Source: CAD feature listing. Evaluate the final solid. Frame: model axes, mm. A direction names the side the tool comes from. Round coordinates to 2 decimals unless told otherwise and drop trailing zeros. Order: outer loops, then holes, each group sorted by start corner. A loop starts at its lowest first (then second) coordinate and runs counter-clockwise, first axis right, second up. Notation, with made-up numbers: M -40,32.25 L -31,32.25 A18 cw -31,56.25 Z; hole C 81,45.25 d7. An arc over 180 degrees is marked long. Answer in a Markdown table with one row per item. Add a question column.
```python
from build123d import *

# Parameters (mm, degrees)
SKETCH1_W                     = 28.2
SKETCH1_H                     = 28.2
BOSS_EXTRUDE1_DEPTH           = 49
SKETCH2_R                     = 11
BOSS_EXTRUDE2_DEPTH           = 2
SKETCH3_R                     = 2.5
BOSS_EXTRUDE3_DEPTH           = 18
FILLET1_R                     = 2
TAP_DRILL_FOR_M2_5_TAP1_D     = 2.05
TAP_DRILL_FOR_M2_5_TAP1_DEPTH = 4.5
TAP_DRILL_FOR_M2_5_TAP1_TIP   = 0.615882135
FILLET2_R                     = 1


with BuildPart() as part:
    # Sketch1 → Boss-Extrude1 (new body)
    with BuildSketch(Plane(origin=(0, 0, 0), x_dir=(1, 0, 0), z_dir=(0, 1, 0))):
        with Locations((14.1, 14.1)):
            Rectangle(SKETCH1_W, SKETCH1_H)
    extrude(amount=BOSS_EXTRUDE1_DEPTH)

    # Sketch2 → Boss-Extrude2 (add)
    with BuildSketch(Plane(origin=(0, 49, 0), x_dir=(1, 0, 0), z_dir=(0, 1, 0))):
        with Locations(Location((14.1, 14.1, 0), (0, 0, 270))):
            Circle(SKETCH2_R)
    extrude(amount=BOSS_EXTRUDE2_DEPTH)

    # Sketch3 → Boss-Extrude3 (add)
    with BuildSketch(Plane(origin=(0, 51, 0), x_dir=(1, 0, 0), z_dir=(0, 1, 0))):
        with Locations(Location((14.1, 14.1, 0), (0, 0, 270))):
            Circle(SKETCH3_R)
    extrude(amount=BOSS_EXTRUDE3_DEPTH)

    # Fillet1
    fillet1_edges = [part.edges().sort_by_distance(p)[0] for p in [
        (0, 24.5, -28.2),
        (28.2, 24.5, -28.2),
        (28.2, 24.5, 0),
        (0, 24.5, 0),
    ]]
    fillet(fillet1_edges, radius=FILLET1_R)

    # Tap Drill for M2.5 Tap1
    with Locations(Plane(origin=(0, 49, 0), x_dir=(1, 0, 0), z_dir=(0, 1, 0))):
        with Locations((2.6, 2.6), (25.6, 2.6), (25.6, 25.6), (2.6, 25.6)):
            Hole(TAP_DRILL_FOR_M2_5_TAP1_D / 2, depth=TAP_DRILL_FOR_M2_5_TAP1_DEPTH)
            with Locations((0, 0, -(TAP_DRILL_FOR_M2_5_TAP1_DEPTH + TAP_DRILL_FOR_M2_5_TAP1_TIP / 2))):  # 118° drill point
                Cone(0, TAP_DRILL_FOR_M2_5_TAP1_D / 2, TAP_DRILL_FOR_M2_5_TAP1_TIP, mode=Mode.SUBTRACT)

    # Fillet2
    fillet2_edges = [part.edges().sort_by_distance(p)[0] for p in [
        (14.1, 0, -28.2),
        (0, 0, -14.1),
        (28.2, 0, -14.1),
        (14.1, 0, 0),
        (0.585786438, 0, -0.585786438),
        (27.614213562, 0, -0.585786438),
        (0.585786438, 0, -27.614213562),
        (27.614213562, 0, -27.614213562),
    ]]
    fillet(fillet2_edges, radius=FILLET2_R)


solid = part.part
```
(1) Cut plane A-A (z = -14.1). Return loops of the section in (x, y), and give its area (3 significant figures).
(2) Pin query (flat end, axial travel): pin 1 (2.5 mm diameter, centred on x = 2.6, z = -2.6, fed in from +Y). Return the tip coordinate at first contact, or that it passes through.
(3) Draft query along X for faces 3 (the face through (0.57, 25.34, -0.6)), 4 (the face through (27.6, 25.34, -27.63)), 5 (the face through (24.65, 46.72, -25.21)). Return one class per face: +X half, -X half, draft (parallel to the pull), parting line (faces both ways), or undercut.
(4) Cut plane B-B (x = 6). Return loops of the section in (y, z), and give its area (3 significant figures).
(5) Cut plane C-C (y = 58.5). Return loops of the section in (x, z), and give its area (3 significant figures).
(6) Cut plane D-D (z = -21). Return loops of the section in (x, y).
(7) Access query for faces 1 (the face through (28.2, 25, -14)), 2 (the face through (8, 49, -24)). Directions: +Z, -Z, +X, -X, +Y, -Y. A direction counts if a zero-diameter tool reaches every point of the face in a straight line with its end or side. Return the directions, or none.
(8) Line query: line 1 (Z direction, x = 2.6, y = 47.25) (3 decimals); line 2 (X direction, y = 47.7, z = -25.6) (3 decimals); line 3 (Y direction, x = 14.5, z = -26.75). Output: solid intervals per line, ascending. Write a range as from..to.
Answer list:
| question | item | result |
|---|---|---|
| 1 | outline | M 0,1 A1 ccw 1,0 L 27.2,0 A1 ccw 28.2,1 L 28.2,49 L 25.1,49 L 25.1,51 L 16.6,51 L 16.6,69 L 11.6,69 L 11.6,51 L 3.1,51 L 3.1,49 L 0,49 Z |
| 1 | area | 1,520 mm² |
| 2 | pin 1 | y = 49 |
| 3 | face 3 | -X half |
| 3 | face 4 | +X half |
| 3 | face 5 | undercut |
| 4 | outline | M 0,-27.2 A1 ccw 1,-28.2 L 49,-28.2 L 49,-21.54 L 51,-21.54 L 51,-6.66 L 49,-6.66 L 49,0 L 1,0 A1 ccw 0,-1 Z |
| 4 | area | 1,410 mm² |
| 5 | outline | C 14.1,-14.1 d5 |
| 5 | area | 19.6 mm² |
| 6 | outline | M 0,1 A1 ccw 1,0 L 27.2,0 A1 ccw 28.2,1 L 28.2,49 L 22.67,49 L 22.67,51 L 5.53,51 L 5.53,49 L 0,49 Z |
| 7 | face 1 | +Z, -Z, +X, +Y, -Y |
| 7 | face 2 | +Y |
| 8 | line 1 | -28.2..-26.625, -24.575..-3.625, -1.575..0 |
| 8 | line 2 | 0..1.575, 3.625..24.575, 26.625..28.2 |
| 8 | line 3 | 0..49 |
